Build history of the part. All positions in model axes, mm. Face numbers are marked on the shaded views. Coordinates: 2 decimals unless noted, no trailing zeros. Write each loop counter-clockwise with the first axis right and the second up, starting at its lowest first coordinate (ties: lowest second). Pieces come first, ordered by that corner, then holes. Notation, with made-up numbers: (-39, 79.5) -> (-33, 79.5) arc R34 cw to (-33, 114.5) -> close; hole circle Ø9 at (-38, 19). An arc over 180 degrees is marked (long way). Write each question's results on one line, items separated by ' | '. Start each with the question number.
Q1. Saw through at C-C on x = 14. Give the cut face in (y, z).
Q2. Saw through at A-A on z = 0. Give the cut face in (x, y).
Q3. Two-plate mould, pull along Z, no slides. Class the marked faces 1, 2, 3 and 4: released by +Z, released by -Z, zero draft, split by the parting line, or undercut.
Q4. Drop a flat-ended pin along its axis: pin 1 Ø6 at (x, z) = (14, 0) entering from +Y. Give the stop position or say it passes through.
Q5. Drill centre lines: line 1 (Z direction, x = 14, y = 3.3); line 2 (X direction, y = 3.3, z = 1); line 3 (X direction, y = 2.1, z = -2.75). Where is each one in solid material? Low to high.
Q6. Saw through at B-B on y = 2.75. Give the cut face in (x, z), and give its area (3 significant figures).
from build123d import *

# Parameters (mm, degrees)
SKETCH1_W            = 40
SKETCH1_H            = 20
BOSS_EXTRUDE1_DEPTH  = 5
M6_CLEARANCE_HOLE1_D = 6.4
FILLET1_R            = 5
CHAMFER1_SIZE        = 0.5


with BuildPart() as part:
    # Sketch1 → Boss-Extrude1 (new body)
    with BuildSketch(Plane(origin=(0, 0, 0), x_dir=(1, 0, 0), z_dir=(0, 1, 0))):
        Rectangle(SKETCH1_W, SKETCH1_H)
    extrude(amount=BOSS_EXTRUDE1_DEPTH)

    # M6 Clearance Hole1 (through all)
    with Locations(Plane(origin=(0, 5, 0), x_dir=(1, 0, 0), z_dir=(0, 1, 0))):
        with Locations((-14, 0), (14, 0)):
            Hole(M6_CLEARANCE_HOLE1_D / 2)

    # Fillet1
    fillet1_edges = [part.edges().sort_by_distance(p)[0] for p in [
        (-20, 2.5, -10),
        (20, 2.5, -10),
    ]]
    fillet(fillet1_edges, radius=FILLET1_R)

    # Chamfer1
    chamfer1_edges = [part.edges().sort_by_distance(p)[0] for p in [
        (0, 5, 10),
        (-20, 0, 2.5),
        (-20, 5, 2.5),
        (0, 0, -10),
        (18.535533906, 0, -8.535533906),
        (-18.535533906, 0, -8.535533906),
        (0, 5, -10),
        (18.535533906, 5, -8.535533906),
        (-18.535533906, 5, -8.535533906),
        (20, 5, 2.5),
        (0, 0, 10),
        (20, 0, 2.5),
        (20, 2.5, 10),
        (-20, 2.5, 10),
    ]]
    chamfer(chamfer1_edges, length=CHAMFER1_SIZE)


solid = part.part
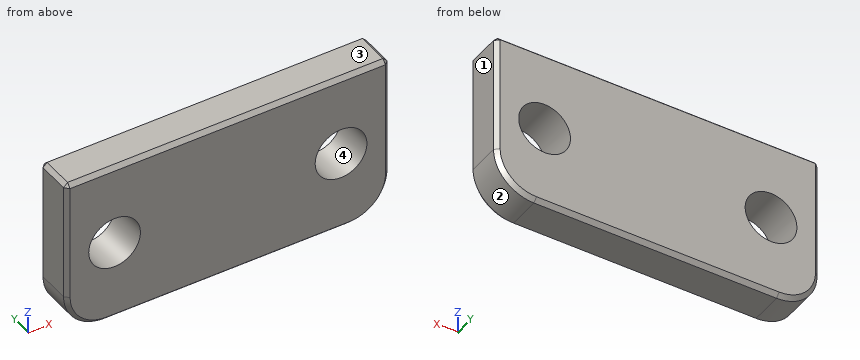
Returned:
1) outline: (0, -9.5) -> (0.5, -10) -> (4.5, -10) -> (5, -9.5) -> (5, -3.2) -> (0, -3.2) -> close; (0, 3.2) -> (5, 3.2) -> (5, 9.5) -> (4.5, 10) -> (0.5, 10) -> (0, 9.5) -> close
2) outline: (-20, 0.5) -> (-19.5, 0) -> (-17.2, 0) -> (-17.2, 5) -> (-19.5, 5) -> (-20, 4.5) -> close; (-10.8, 0) -> (10.8, 0) -> (10.8, 5) -> (-10.8, 5) -> close; (17.2, 0) -> (19.5, 0) -> (20, 0.5) -> (20, 4.5) -> (19.5, 5) -> (17.2, 5) -> close
3) face 1: zero draft | face 2: released by -Z | face 3: released by +Z | face 4: undercut
4) pin 1: passes through
5) line 1: z = -10 to -3.2, 3.2 to 10 | line 2: x = -20 to -17.04, -10.96 to 10.96, 17.04 to 20 | line 3: x = -20 to -15.64, -12.36 to 12.36, 15.64 to 20
6) outline: (-20, -5) arc R5 ccw to (-15, -10) -> (15, -10) arc R5 ccw to (20, -5) -> (20, 9.5) -> (19.5, 10) -> (-19.5, 10) -> (-20, 9.5) -> close; hole circle Ø6.4 at (-14, 0); hole circle Ø6.4 at (14, 0) | area: 725 mm2
